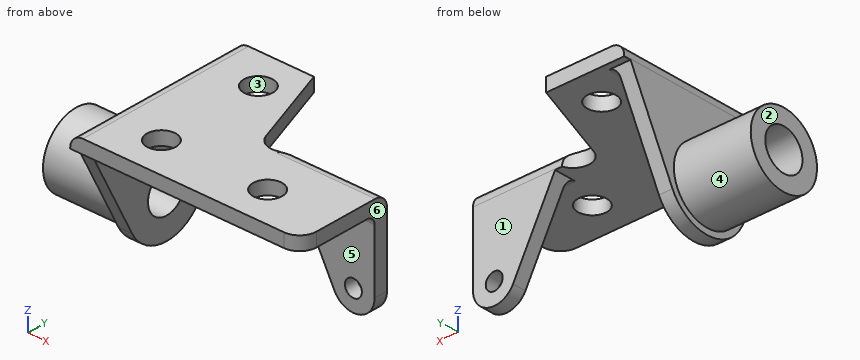
from build123d import *

# Parameters (mm, degrees)
SKETCH1_R           = 2.159
BOSS_EXTRUDE1_DEPTH = 2.032
BOSS_EXTRUDE2_DEPTH = 2.032
SKETCH3_R           = 5.4356
BOSS_EXTRUDE3_DEPTH = 11.5
SKETCH4_R           = 3.048
CUT_EXTRUDE1_DEPTH  = 57.097468274
SKETCH5_R           = 1.27
BOSS_EXTRUDE4_DEPTH = 2.032
CUT_EXTRUDE2_DEPTH  = 14.732
FILLET4_R           = 1.905
FILLET5_R           = 1.27
FILLET6_R           = 2.54


with BuildPart() as part:
    # Sketch1 → Boss-Extrude1 (new body)
    with BuildSketch(Plane.XY):
        with BuildLine():
            Line((0, 0), (0, 27.1526))
            Line((0, 27.1526), (11.684, 27.1526))
            Line((11.684, 27.1526), (16.440472212, 14.0843))
            ThreePointArc((16.440472212, 14.0843), (18.827291469, 12.413031164), (21.214110726, 14.0843))
            Line((21.214110726, 14.0843), (34.544, 14.0843))
            Line((34.544, 14.0843), (34.544, 0))
            Line((34.544, 0), (0, 0))
        make_face()
        with Locations((8.509, 21.5265)):
            Circle(SKETCH1_R, mode=Mode.SUBTRACT)
        with Locations((8.509, 5.6261)):
            Circle(SKETCH1_R, mode=Mode.SUBTRACT)
        with Locations((24.4094, 5.6261)):
            Circle(SKETCH1_R, mode=Mode.SUBTRACT)
    extrude(amount=BOSS_EXTRUDE1_DEPTH)

    # Sketch2 → Boss-Extrude2 (add)
    with BuildSketch(Plane.ZY):
        with BuildLine():
            Line((2.032, 0), (-13.544651807, 7.915259956))
            ThreePointArc((-13.544651807, 7.915259956), (-17.018, 13.5763), (-13.544651807, 19.237340044))
            Line((-13.544651807, 19.237340044), (2.032, 27.1526))
            Line((2.032, 27.1526), (2.032, 0))
        make_face()
    extrude(amount=-BOSS_EXTRUDE2_DEPTH)

    # Sketch3 → Boss-Extrude3 (add)
    with BuildSketch(Plane.ZY):
        with Locations(Location((-10.668, 13.5763, 0), (0, 0, 180))):
            Circle(SKETCH3_R)
    extrude(amount=BOSS_EXTRUDE3_DEPTH)

    # Sketch4 → Cut-Extrude1 (cut, through all)
    with BuildSketch(Plane.ZY.offset(11.5)):
        with Locations((-10.668, 13.5763)):
            Circle(SKETCH4_R)
    extrude(amount=-CUT_EXTRUDE1_DEPTH, mode=Mode.SUBTRACT)

    # Sketch5 → Boss-Extrude4 (add)
    with BuildSketch(Plane(origin=(0, 14.0843, 0), x_dir=(1, 0, 0), z_dir=(0, 1, 0))):
        with BuildLine():
            Line((21.214110726, -2.032), (28.549831644, 12.128450197))
            ThreePointArc((28.549831644, 12.128450197), (32.120586811, 13.752759677), (34.544, 10.668))
            Line((34.544, 10.668), (34.544, -2.032))
            Line((34.544, -2.032), (21.214110726, -2.032))
        make_face()
        with Locations(Location((31.369, 10.668, 0), (0, 0, 270))):
            Circle(SKETCH5_R, mode=Mode.SUBTRACT)
    extrude(amount=-BOSS_EXTRUDE4_DEPTH)

    # Sketch6 → Cut-Extrude2 (cut)
    with BuildSketch(Plane(origin=(34.544, 0, 0), x_dir=(0, 0, -1), z_dir=(1, 0, 0))):
        with BuildLine():
            Line((-0.127, 14.0843), (-2.032, 14.0843))
            Line((-2.032, 14.0843), (-2.032, 12.1793))
            ThreePointArc((-2.032, 12.1793), (-1.474038418, 13.526338418), (-0.127, 14.0843))
        make_face()
    extrude(amount=-CUT_EXTRUDE2_DEPTH, mode=Mode.SUBTRACT)

    # Fillet4
    fillet4_edges = [part.edges().sort_by_distance(p)[0] for p in [
        (0, 13.5763, 2.032),
    ]]
    fillet(fillet4_edges, radius=FILLET4_R)

    # Fillet5
    fillet5_edges = [part.edges().sort_by_distance(p)[0] for p in [
        (2.032, 13.5763, 0),
        (28.405386966, 12.0523, 0),
    ]]
    fillet(fillet5_edges, radius=FILLET5_R)

    # Fillet6
    fillet6_edges = [part.edges().sort_by_distance(p)[0] for p in [
        (34.544, 0, 1.016),
    ]]
    fillet(fillet6_edges, radius=FILLET6_R)


solid = part.part
Can you work these out from the model? Positions are in its coordinate system, mm. Face numbers are marked on the shaded views. A direction names the side the tool comes from. Give positions to 0.01 mm unless a question says otherwise; leave off trailing zeros. Loops run counter-clockwise (first coordinate to the right, second up) from the corner with the lowest first, then second, coordinate; pieces in that order, holes last. Notation, with made-up numbers: (74.5, 29) -> (117.5, 29) arc R25 cw to (117.5, 47) -> close; hole circle Ø2 at (84.5, -21.5). An arc over 180 degrees is marked (long way). Use one line per item in the form item = value.
1) If we section it at A-A (y = 7): Please give me the cut outline in (x, z) (3 decimals).
Answers:
outline = (0, -11.743) -> (2.032, -11.743) -> (2.032, -1.27) arc R1.27 cw to (3.302, 0) -> (6.844, 0) -> (6.844, 2.032) -> (1.905, 2.032) arc R1.905 ccw to (0, 0.127) -> close; (10.174, 0) -> (22.744, 0) -> (22.744, 2.032) -> (10.174, 2.032) -> close; (26.075, 0) -> (34.544, 0) -> (34.544, 2.032) -> (26.075, 2.032) -> close
2) If we section it at B-B (z = -3.75): Please give me the cut outline in (x, y), plus the area to 3 significant figures.
Answers:
outline = (0, 2.94) -> (2.03, 2.94) -> (2.03, 24.21) -> (0, 24.21) -> close; (24.21, 12.05) -> (34.54, 12.05) -> (34.54, 14.08) -> (24.21, 14.08) -> close
area = 64.2 mm²
3) I need wall thicknesses on line 1 along Z through (x, y) = (12.5, 12); line 2 along X through (y, z) = (10, -12.5). Which ranges of each line are inside material? Lowest first, please.
Answers:
line_1 = 0 to 2.03
line_2 = -11.5 to 2.03
4) If we section it at C-C (x = 7.5): Please give me the cut outline in (y, z).
Answers:
outline = (0, 0) -> (3.72, 0) -> (3.72, 2.03) -> (0, 2.03) -> close; (7.53, 0) -> (19.62, 0) -> (19.62, 2.03) -> (7.53, 2.03) -> close; (23.44, 0) -> (27.15, 0) -> (27.15, 2.03) -> (23.44, 2.03) -> close
5) For the marked faces 4, 5 and 6, which set-ups out of +Z, -Z, +X, -X, +Y, -Y let a thin tool reach every point of the face, with its end or its side?
Answers:
face_4 = -X
face_5 = -Z, +X, -Y
face_6 = +Z, -Z, +X, +Y, -Y
6) If we section it at D-D (z = -14.5): Please give me the cut outline in (x, y), plus the area to 3 significant figures.
Answers:
outline = (-11.5, 9.72) -> (0, 9.72) -> (0, 8.51) -> (2.03, 8.51) -> (2.03, 18.64) -> (0, 18.64) -> (0, 17.43) -> (-11.5, 17.43) -> close
area = 109 mm²
7) We'd pull the mould along X, two halves only. Please class the marked faces 1, 2 and 3: released by +X, released by -X, zero draft, split by the parting line, or undercut.
Answers:
face_1 = zero draft
face_2 = released by -X
face_3 = undercut
8) Will these pins go through, and if not, where does the flat tip stop? pin 1 (5 mm diameter, centred on x = 8.51, y = 5.63, fed in from -Z); pin 2 (6 mm diameter, centred on x = 27, z = -5, fed in from -Y); pin 3 (10 mm diameter, centred on y = 23.5, z = -6, fed in from -X).
Answers:
pin_1 = 0
pin_2 = 12.05
pin_3 = 0
